Work out the finished part from the listing and answer in its coordinate system (mm). Give positions to 0.01 mm unless a question says otherwise; leave off trailing zeros. Loops run counter-clockwise (first coordinate to the right, second up) from the corner with the lowest first, then second, coordinate; pieces in that order, holes last. Notation, with made-up numbers: M -17.5,76.25 L 6.5,76.25 A32 cw 6.5,113.25 Z; hole C 74,26.25 d4. An arc over 180 degrees is marked long. Answer in a Markdown table with one row per item. Add a question column.
from build123d import *

# Parameters (mm, degrees)
SKETCH1_R           = 5
BOSS_EXTRUDE1_DEPTH = 8
CHAMFER1_SIZE       = 1
SKETCH2_OUTSIDE_W   = 54.734
SKETCH2_OUTSIDE_H   = 57.674
SKETCH2_OUTSIDE_R   = 9.5
CUT_EXTRUDE1_DEPTH  = 8
CUT_EXTRUDE1_DRAFT  = -60
SKETCH3_OUTSIDE_W   = 54.734
SKETCH3_OUTSIDE_H   = 57.674
SKETCH3_OUTSIDE_R   = 9.5
CUT_EXTRUDE2_DEPTH  = 8
CUT_EXTRUDE2_DRAFT  = -60


with BuildPart() as part:
    # Sketch1 → Boss-Extrude1 (new body)
    with BuildSketch(Plane(origin=(0, 0, 0), x_dir=(1, 0, 0), z_dir=(0, 1, 0))):
        Polygon((9.5, -5.484827557), (9.5, 5.484827557), (0, 10.969655115), (-9.5, 5.484827557), (-9.5, -5.484827557), (0, -10.969655115), align=None)
        with Locations(Location((0, 0, 0), (0, 0, 270))):
            Circle(SKETCH1_R, mode=Mode.SUBTRACT)
    extrude(amount=BOSS_EXTRUDE1_DEPTH)

    # Chamfer1
    chamfer1_edges = [part.edges().sort_by_distance(p)[0] for p in [
        (0, 0, -5),
        (0, 8, -5),
    ]]
    chamfer(chamfer1_edges, length=CHAMFER1_SIZE)


with BuildPart() as cut_extrude1_tool:
    # Sketch2 outside → Cut-Extrude1 (with draft: the straight prism first)
    with BuildSketch(Plane(origin=(0, 8, 0), x_dir=(1, 0, 0), z_dir=(0, 1, 0))):
        Rectangle(SKETCH2_OUTSIDE_W, SKETCH2_OUTSIDE_H)
        Circle(SKETCH2_OUTSIDE_R, mode=Mode.SUBTRACT)
    extrude(amount=-CUT_EXTRUDE1_DEPTH)
    # Cut-Extrude1: the draft: its side faces are tilted about the plane it starts from
    cut_extrude1_sides = [cut_extrude1_tool.faces().sort_by_distance(p)[0] for p in [
        (0, 4, 28.837),
        (27.367, 4, 0),
        (0, 4, -28.837),
        (-27.367, 4, 0),
        (-9.5, 4, 0),
    ]]
    draft(cut_extrude1_sides, Plane(origin=(0, 8, 0), x_dir=(1, 0, 0), z_dir=(0, 1, 0)), CUT_EXTRUDE1_DRAFT)


with BuildPart() as part_1:
    add(part.part)

    # Cut-Extrude1: cut by cut_extrude1_tool
    add(cut_extrude1_tool.part, mode=Mode.SUBTRACT)


with BuildPart() as cut_extrude2_tool:
    # Sketch3 outside → Cut-Extrude2 (with draft: the straight prism first)
    with BuildSketch(Plane.XZ):
        Rectangle(SKETCH3_OUTSIDE_W, SKETCH3_OUTSIDE_H)
        Circle(SKETCH3_OUTSIDE_R, mode=Mode.SUBTRACT)
    extrude(amount=-CUT_EXTRUDE2_DEPTH)
    # Cut-Extrude2: the draft: its side faces are tilted about the plane it starts from
    cut_extrude2_sides = [cut_extrude2_tool.faces().sort_by_distance(p)[0] for p in [
        (0, 4, -28.837),
        (27.367, 4, 0),
        (0, 4, 28.837),
        (-27.367, 4, 0),
        (-9.5, 4, 0),
    ]]
    draft(cut_extrude2_sides, Plane.XZ, CUT_EXTRUDE2_DRAFT)


with BuildPart() as part_2:
    add(part_1.part)

    # Cut-Extrude2: cut by cut_extrude2_tool
    add(cut_extrude2_tool.part, mode=Mode.SUBTRACT)


solid = part_2.part
(1) The mould has two halves that part along Z. Classify faces 1 (the face through (9.5, 4, 0)), 2 (the face through (8.54, 0.2, 4.9)), 3 (the face through (-4.88, 3.96, -1.08)): pulls with the +Z half, pulls with the -Z half, needs draft (parallel to the pull), parting line crosses it, or undercut.
(2) Section A-A, the plane y = 4.25 is taken. Determine the outline of the cut face in (x, z), and give its area (3 significant figures).
(3) Section B-B, the plane y = 7.5 is taken. Determine the outline of the cut face in (x, z), and give its area (3 significant figures).
(4) Consider line 1 along X through (y, z) = (3.45, 0); line 2 along Z through (x, y) = (4.25, 4.25); line 3 along Z through (x, y) = (-0.25, 0.5). Determine where each line is inside the solid, lowest interval first. Write a range as from..to.
(5) Each of these flat-tipped pins is pushed along its axis until it touches: P1, Ø2, axis at y = 2.5, z = 8, coming from the +X side; P2, Ø2, axis at x = -4.5, z = 1.5, coming from the +Y side; P3, Ø1, axis at x = 5.5, z = -5, coming from the -Y side; P4, Ø2, axis at x = -6.5, y = 2.5, coming from the +Z side. Where does it stop, or does it pass through?
Numbers:
| question | item | result |
|---|---|---|
| 1 | face 1 | needs draft |
| 1 | face 2 | pulls with the +Z half |
| 1 | face 3 | undercut |
| 2 | outline | M -9.5,-5.48 L 0,-10.97 L 9.5,-5.48 L 9.5,5.48 L 0,10.97 L -9.5,5.48 Z; hole C 0,0 d10 |
| 2 | area | 234 mm² |
| 3 | outline | M -9.5,-4.15 A10.37 ccw -8.34,-6.15 L -1.16,-10.3 A10.37 ccw 1.16,-10.3 L 8.34,-6.15 A10.37 ccw 9.5,-4.15 L 9.5,4.15 A10.37 ccw 8.34,6.15 L 1.16,10.3 A10.37 ccw -1.16,10.3 L -8.34,6.15 A10.37 ccw -9.5,4.15 Z; hole C 0,0 d11 |
| 3 | area | 214 mm² |
| 4 | line 1 | x = -9.5..-5, 5..9.5 |
| 4 | line 2 | z = -8.52..-2.63, 2.63..8.52 |
| 4 | line 3 | z = -10.36..-5.49, 5.49..10.36 |
| 5 | P1 | stops at x = 6.88 |
| 5 | P2 | stops at y = 7.74 |
| 5 | P3 | stops at y = 0 |
| 5 | P4 | stops at z = 7.79 |
